from build123d import *

# Parameters (mm, degrees)
SKETCH1_W           = 36
SKETCH1_H           = 30
BOSS_EXTRUDE1_DEPTH = 6.5
SKETCH2_R           = 3.175
CUT_EXTRUDE1_DEPTH  = 5
SKETCH3_RX          = 4.5
SKETCH3_RY          = 3.5
CUT_EXTRUDE3_DEPTH  = 30


with BuildPart() as part:
    # Sketch1 → Boss-Extrude1 (new body)
    with BuildSketch(Plane(origin=(0, 0, 0), x_dir=(1, 0, 0), z_dir=(0, 1, 0))):
        with Locations((-18, -15)):
            Rectangle(SKETCH1_W, SKETCH1_H)
    extrude(amount=BOSS_EXTRUDE1_DEPTH)

    # Sketch2 → Cut-Extrude1 (cut)
    with BuildSketch(Plane(origin=(0, 6.5, 0), x_dir=(1, 0, 0), z_dir=(0, 1, 0))):
        with Locations((-18, -15)):
            Circle(SKETCH2_R)
    extrude(amount=-CUT_EXTRUDE1_DEPTH, mode=Mode.SUBTRACT)

    # Sketch3 → Cut-Extrude3 (cut)
    with BuildSketch(Plane.XY.offset(30)):
        with Locations(Location((-7.4125, 6.5), (0, 0, -180))):
            Ellipse(SKETCH3_RX, SKETCH3_RY)
        with Locations(Location((-28.5875, 6.5), (0, 0, 0))):
            Ellipse(SKETCH3_RX, SKETCH3_RY)
    extrude(amount=-CUT_EXTRUDE3_DEPTH, mode=Mode.SUBTRACT)


solid = part.part
Verification items for the finished model (mm, model axes). A direction names the side the tool comes from. Coordinates: 2 decimals unless noted, no trailing zeros. Order: outer loops, then holes, each group sorted by start corner. A loop starts at its lowest first (then second) coordinate and runs counter-clockwise, first axis right, second up. Notation, with made-up numbers: M 76.25,32.5 L 92.25,32.5 A23 cw 92.25,44.5 Z; hole C 87,11 d4. An arc over 180 degrees is marked long. Return JSON: item names as keys, results as strings.
1) Cross-section at A-A, the plane x = -18. Record the boundary of the cut face in (y, z) (3 decimals), and give its area (3 significant figures).
Answer list:
{"outline": "M 0,0 L 6.5,0 L 6.5,11.825 L 1.5,11.825 L 1.5,18.175 L 6.5,18.175 L 6.5,30 L 0,30 Z", "area": "163 mm2"}
2) Thickness scan on L1, parallel to Z at x = -18, y = 4.4 (3 decimals); L2, parallel to X at y = 4.25, z = 15 (3 decimals); L3, parallel to X at y = 2.9, z = 15 (3 decimals). Record the ranges inside material, lowest first. Write a range as [from, to].
Answer list:
{"L1": "[0, 11.825], [18.175, 30]", "L2": "[-36, -32.034], [-25.141, -21.175], [-14.825, -10.859], [-3.966, 0]", "L3": "[-36, -21.175], [-14.825, 0]"}
3) Cross-section at C-C, the plane y = 4.5. Count the separate pieces of the cut face and the enclosed holes in it, and give its area (3 significant figures).
Answer list:
{"separate pieces": "3", "enclosed holes": "1", "area": "605 mm2"}
4) Cross-section at B-B, the plane y = 2.5. Record the boundary of the cut face in (x, z) (3 decimals), and give its area (3 significant figures).
Answer list:
{"outline": "M -36,0 L 0,0 L 0,30 L -36,30 Z; hole C -18,15 d6.35", "area": "1,050 mm2"}
5) Release check for a two-part mould opening along X. For faces 3 (the flat face through (-36, 3, 15)), 4 (the flat face through (-1, 6.5, 15)), 5 (the flat face through (-18, 1.5, 15)) record: +X half, -X half, draft (parallel to the pull), parting line (faces both ways), or undercut.
Answer list:
{"face 3": "-X half", "face 4": "draft", "face 5": "undercut"}
6) Gauge pin test, flat end, axial feed: pin 1 (1 mm diameter, centred on x = -8, z = 22, fed in from -Y). Record the tip position at first contact, or that the pin passes through.
Answer list:
{"pin 1": "y = 0"}
7) Access from +Z, -Z, +X, -X, +Y, -Y to the whole of each face (thin tool, end or side, straight path). Record for faces 1 (the cylindrical face through (-21.17, 4.04, 14.86)), 2 (the flat face through (-35, 6.5, 15)).
Answer list:
{"face 1": "+Y", "face 2": "+Z, -Z, +X, -X, +Y"}
